Design review of the part built by this model. Coordinates are the model's own, in mm. Coordinates: 2 decimals unless noted, no trailing zeros. Order: outer loops, then holes, each group sorted by start corner. A loop starts at its lowest first (then second) coordinate and runs counter-clockwise, first axis right, second up. Notation, with made-up numbers: M 9,60 L 41,60 A20 ccw 41,83 Z; hole C -32,79.5 d1. An arc over 180 degrees is marked long. Answer as a JSON object with one key per item and string values.
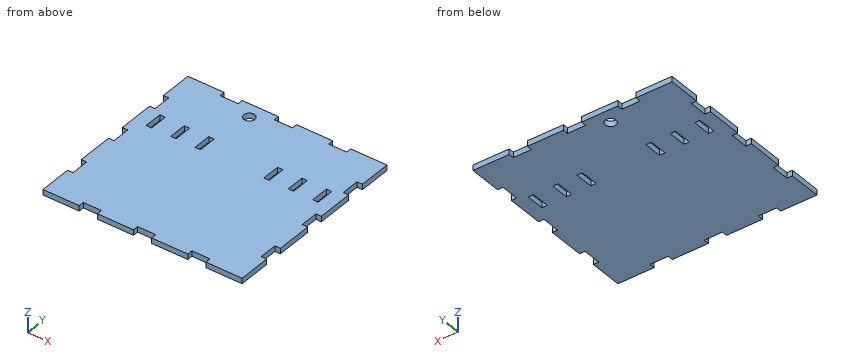
from build123d import *

# Parameters (mm, degrees)
F1_DEPTH = 3
F2_W     = 2.98
F2_H     = 10
F3_DEPTH = 25
F4_R     = 3
F5_DEPTH = 25


with BuildPart() as f1:
    # F0 (on Top) → F1 (new body)
    with BuildSketch(Plane.XY):
        Polygon((35, -53), (55, -53), (55, -35), (52, -35), (52, -25), (55, -25), (55, -5), (52, -5), (52, 5), (55, 5), (55, 25), (52, 25), (52, 35), (55, 35), (55, 53), (35, 53), (35, 52), (35, 50), (25, 50), (25, 52), (25, 53), (5, 53), (5, 52), (5, 50), (-5, 50), (-5, 52), (-5, 53), (-25, 53), (-25, 52), (-25, 50), (-35, 50), (-35, 52), (-35, 53), (-55, 53), (-55, 35), (-52, 35), (-52, 25), (-55, 25), (-55, 5), (-52, 5), (-52, -5), (-55, -5), (-55, -25), (-52, -25), (-52, -35), (-55, -35), (-55, -53), (-35, -53), (-35, -52), (-35, -50), (-25, -50), (-25, -52), (-25, -53), (-5, -53), (-5, -52), (-5, -50), (5, -50), (5, -52), (5, -53), (25, -53), (25, -52), (25, -50), (35, -50), (35, -52), align=None)
    extrude(amount=F1_DEPTH)

    # F2 (on face) → F3 (cut)
    with BuildSketch(Plane(origin=(0, 0, 0), x_dir=(1, 0, 0), z_dir=(0, 0, -1))):
        with Locations((-46.01, -17.55)):
            Rectangle(F2_W, F2_H)
        with Locations((-32.5, -17.55)):
            Rectangle(F2_W, F2_H)
        with Locations((-18.99, -17.55)):
            Rectangle(F2_W, F2_H)
        with Locations((18.99, -17.55)):
            Rectangle(F2_W, F2_H)
        with Locations((32.5, -17.55)):
            Rectangle(F2_W, F2_H)
        with Locations((46.01, -17.55)):
            Rectangle(F2_W, F2_H)
    extrude(amount=-F3_DEPTH, mode=Mode.SUBTRACT)

    # F4 (on face) → F5 (cut)
    with BuildSketch(Plane.XY.offset(3)):
        with Locations((-15, 45)):
            Circle(F4_R)
    extrude(amount=-F5_DEPTH, mode=Mode.SUBTRACT)


solid = f1.part
1) Add section D-D (y = 27). State the section outline as (x, z) points.
Taken from the geometry:
{"outline": "M -52,0 L 52,0 L 52,3 L -52,3 Z"}
2) Add section A-A (y = 45). State the section outline as (x, z) points.
Taken from the geometry:
{"outline": "M -55,0 L -18,0 L -18,3 L -55,3 Z; M -12,0 L 55,0 L 55,3 L -12,3 Z"}
3) Add section C-C (z = 2.25). Count the separate pieces of the cut face and the enclosed holes in it, and give its area (3 significant figures).
Taken from the geometry:
{"separate pieces": "1", "enclosed holes": "7", "area": "11,100 mm2"}
4) Add section B-B (x = -15). State the section outline as (y, z) points, and give its area (3 significant figures).
Taken from the geometry:
{"outline": "M -53,0 L 42,0 L 42,3 L -53,3 Z; M 48,0 L 53,0 L 53,3 L 48,3 Z", "area": "300 mm2"}
5) To check wall thickness, follow L1, parallel to Y at x = -19.5, z = 2.65; L2, parallel to Y at x = -15, z = 0.6; L3, parallel to X at y = 30.5, z = 2.75. State the ranges of each line that lie inside material, in increasing order.
Taken from the geometry:
{"L1": "y = -53 to 12.55, 22.55 to 53", "L2": "y = -53 to 42, 48 to 53", "L3": "x = -52 to 52"}
6) Insertion check: pin 1 Ø0.9 at (x, z) = (-31, 1) entering from -Y; pin 2 Ø1 at (y, z) = (-32.5, 0.5) entering from +X. Each pin has a flat end and moves straight along its axis. Give the tip position at first contact, or say it passes through.
Taken from the geometry:
{"pin 1": "stops at y = -50", "pin 2": "stops at x = 52"}
